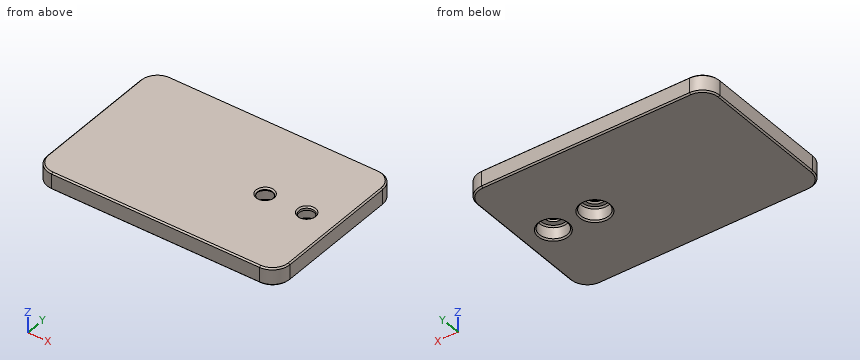
Autodesk Inventor part; units mm, degrees
ref_plane "YZ Plane" through (0, 0, 0) normal (1, 0, 0) x (0, 1, 0)
ref_plane "XZ Plane" through (0, 0, 0) normal (0, 1, 0) x (-1, 0, 0)
ref_plane "XY Plane" through (0, 0, 0) normal (0, 0, 1) x (1, 0, 0)
sketch "Sketch1" plane through (0, 0, 0) normal (0, 0, 1) x (1, 0, 0)
  line L0 (-35, 23) -> (35, 23)
  line L1 (35, 23) -> (35, -23)
  line L2 (35, -23) -> (-35, -23)
  line L3 (-35, -23) -> (-35, 23)
  point P0 (0, 0)
  point P1 (0, 23)
  point P2 (35, 0)
  dimension "d0" = 46
  dimension "d1" = 70
extrude "Extrusion1" add sketch "Sketch1" along normal blind 5
sketch "Sketch3" plane through (0, 0, 0) normal (0, 0, -1) x (-1, 0, 0)
  line L0 (-26.46, 0) -> (-14.46, 0) construction
  line L1 (-35, -23) -> (-35, 23)
  point P0 (0, 0)
  dimension "d7" = 12
  dimension "d8" = 8.54
hole "Hole1" at (14.46, 0, 0) at (26.46, 0, 0) direction (0, 0, 1) diameter 4.4 end through all counterbore diameter 8 counterbore depth 4
fillet "Fillet1" radius 5 4 edges at (35, -23, 2.5) (35, 23, 2.5) (-35, 23, 2.5) (-35, -23, 2.5)
chamfer "Chamfer2" distance 0.4 angle 45 23 edges at (0, -23, 5) (33.5355, -21.5355, 5) (35, 0, 5) (33.5355, 21.5355, 5) (0, 23, 5) (-33.5355, 21.5355, 5) (-35, 0, 5) (-33.5355, -21.5355, 5) (0, -23, 0) (33.5355, -21.5355, 0) (35, 0, 0) (33.5355, 21.5355, 0) (0, 23, 0) (-33.5355, 21.5355, 0) (-35, 0, 0) (-33.5355, -21.5355, 0) (14.46, -4, 0) (26.46, -4, 0) (26.46, -2.2, 5) (14.46, -2.2, 5) (14.46, -2.2, 4) (14.46, -4, 4) (26.46, -4, 4)
equation "\"d2\" = thickness"
equation "\"thickness\" = 5"
properties part number "Takumar-foot-flat"
Could you check a few things on this model? Use its own coordinates, in mm. Give positions to 0.01 mm unless a question says otherwise; leave off trailing zeros. Order: outer loops, then holes, each group sorted by start corner. A loop starts at its lowest first (then second) coordinate and runs counter-clockwise, first axis right, second up. Notation, with made-up numbers: (10, 65) - (56, 65) arc R6 cw to (56, 71) - close; hole circle Ø6 at (49, 37.25). An arc over 180 degrees is marked (long way). One line per item, written item: value. Start each with the question number.
1. For P1, Ø3.5, axis at x = 13.5, y = -1.5, coming from the -Z side, with a flat end and sliding along its axis, tell me the tip position at first contact or that it passes through.
2. Imagine slicing it at C-C on x = 14.46. List the corners of the cut face in (y, z) for me, plus the area to 3 significant figures.
3. Imagine slicing it at B-B on z = 2.85. List the corners of the cut face in (x, y) for me.
4. Imagine slicing it at D-D on y = 0. Give the number of separate pieces and of enclosed holes in the cut face, plus the area to 3 significant figures.
5. Imagine slicing it at A-A on x = 26.46. List the corners of the cut face in (y, z) for me.
6. If I drill on probe 1 along Y at (x, z) = (26.46, 1.4); probe 2 along X at (y, z) = (0, 4.5); probe 3 along Y at (x, z) = (14.46, 4.5), over which ranges is the centre line in solid material (lowest first)?
Values:
1. P1: z = 4
2. outline: (-23, 0.4) - (-22.6, 0) - (-4.4, 0) - (-4, 0.4) - (-4, 3.6) - (-3.6, 4) - (-2.6, 4) - (-2.2, 4.4) - (-2.2, 4.6) - (-2.6, 5) - (-22.6, 5) - (-23, 4.6) - close; (2.2, 4.4) - (2.6, 4) - (3.6, 4) - (4, 3.6) - (4, 0.4) - (4.4, 0) - (22.6, 0) - (23, 0.4) - (23, 4.6) - (22.6, 5) - (2.6, 5) - (2.2, 4.6) - close
2. area: 193 mm²
3. outline: (-35, -18) arc R5 ccw to (-30, -23) - (30, -23) arc R5 ccw to (35, -18) - (35, 18) arc R5 ccw to (30, 23) - (-30, 23) arc R5 ccw to (-35, 18) - close; hole circle Ø8 at (14.46, 0); hole circle Ø8 at (26.46, 0)
4. separate pieces: 3
4. enclosed holes: 0
4. area: 276 mm²
5. outline: (-23, 0.4) - (-22.6, 0) - (-4.4, 0) - (-4, 0.4) - (-4, 3.6) - (-3.6, 4) - (-2.2, 4) - (-2.2, 4.6) - (-2.6, 5) - (-22.6, 5) - (-23, 4.6) - close; (2.2, 4) - (3.6, 4) - (4, 3.6) - (4, 0.4) - (4.4, 0) - (22.6, 0) - (23, 0.4) - (23, 4.6) - (22.6, 5) - (2.6, 5) - (2.2, 4.6) - close
6. probe 1: -23 to -4, 4 to 23
6. probe 2: -35 to 12.26, 16.66 to 24.26, 28.66 to 35
6. probe 3: -23 to -2.2, 2.2 to 23
